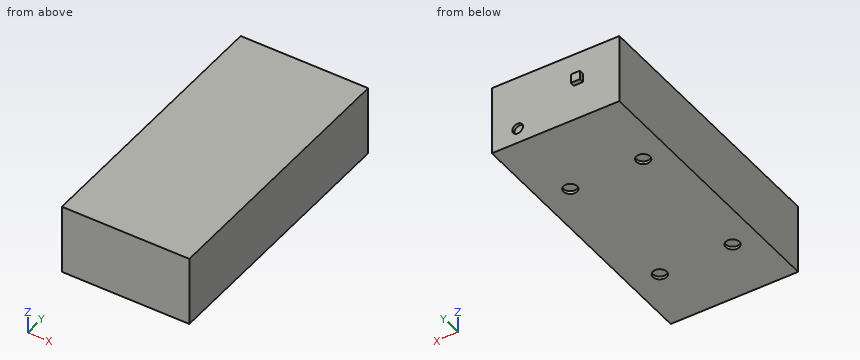
from build123d import *

# Parameters (mm, degrees)
SKETCH1_W           = 90
SKETCH1_H           = 42
SKETCH1_R           = 2.25
BOSS_EXTRUDE1_DEPTH = 23
SKETCH1_3_R         = 2.25
CUT_EXTRUDE1_DEPTH  = 1
SKETCH2_R           = 1.75
CUT_EXTRUDE2_DEPTH  = 1
SKETCH2_3_W         = 3
SKETCH2_3_H         = 3
BOSS_EXTRUDE2_DEPTH = 1.5


with BuildPart() as part:
    # Sketch1 → Boss-Extrude1 (new body)
    # profile 1 of 5: a face of its own
    with BuildSketch(Plane(origin=(0, 0, 0), x_dir=(0, 1, 0), z_dir=(0, 0, 1))):
        Rectangle(SKETCH1_W, SKETCH1_H)
        with Locations((20, 12.5)):
            Circle(SKETCH1_R, mode=Mode.SUBTRACT)
        with Locations((20, -11.5)):
            Circle(SKETCH1_R, mode=Mode.SUBTRACT)
        with Locations((-25, -11.5)):
            Circle(SKETCH1_R, mode=Mode.SUBTRACT)
        with Locations((-25, 12.5)):
            Circle(SKETCH1_R, mode=Mode.SUBTRACT)
    # profile 2 of 5: a face of its own
    with BuildSketch(Plane(origin=(0, 0, 0), x_dir=(0, 1, 0), z_dir=(0, 0, 1))):
        with Locations((-25, -11.5)):
            Circle(SKETCH1_R)
    # profile 3 of 5: a face of its own
    with BuildSketch(Plane(origin=(0, 0, 0), x_dir=(0, 1, 0), z_dir=(0, 0, 1))):
        with Locations((-25, 12.5)):
            Circle(SKETCH1_R)
    # profile 4 of 5: a face of its own
    with BuildSketch(Plane(origin=(0, 0, 0), x_dir=(0, 1, 0), z_dir=(0, 0, 1))):
        with Locations((20, -11.5)):
            Circle(SKETCH1_R)
    # profile 5 of 5: a face of its own
    with BuildSketch(Plane(origin=(0, 0, 0), x_dir=(0, 1, 0), z_dir=(0, 0, 1))):
        with Locations((20, 12.5)):
            Circle(SKETCH1_R)
    extrude(amount=BOSS_EXTRUDE1_DEPTH)

    # Sketch1_3 → Cut-Extrude1 (cut)
    with BuildSketch(Plane(origin=(0, 0, 0), x_dir=(0, 1, 0), z_dir=(0, 0, 1))):
        with Locations(Location((-25, -11.5, 0), (0, 0, 270))):
            Circle(SKETCH1_3_R)
        with Locations(Location((-25, 12.5, 0), (0, 0, 270))):
            Circle(SKETCH1_3_R)
        with Locations(Location((20, -11.5, 0), (0, 0, 270))):
            Circle(SKETCH1_3_R)
        with Locations(Location((20, 12.5, 0), (0, 0, 270))):
            Circle(SKETCH1_3_R)
    extrude(amount=CUT_EXTRUDE1_DEPTH, mode=Mode.SUBTRACT)

    # Sketch2 → Cut-Extrude2 (cut)
    with BuildSketch(Plane(origin=(0, 45, 0), x_dir=(-1, 0, 0), z_dir=(0, 1, 0))):
        with Locations(Location((-12.5, 5, 0), (0, 0, 90))):
            Circle(SKETCH2_R)
    extrude(amount=-CUT_EXTRUDE2_DEPTH, mode=Mode.SUBTRACT)

    # Sketch2_3 → Boss-Extrude2 (add)
    with BuildSketch(Plane(origin=(0, 45, 0), x_dir=(-1, 0, 0), z_dir=(0, 1, 0))):
        with Locations((7.5, 13.5)):
            Rectangle(SKETCH2_3_W, SKETCH2_3_H)
    extrude(amount=BOSS_EXTRUDE2_DEPTH)


solid = part.part
Model file for the job. Use its own axes, mm. Round coordinates to 2 decimals unless told otherwise and drop trailing zeros. Order: outer loops, then holes, each group sorted by start corner. A loop starts at its lowest first (then second) coordinate and runs counter-clockwise, first axis right, second up.
(1) Band-saw the part on B-B (x = -12.5). List the corners of the cut face in (y, z).
(2) Band-saw the part on A-A (z = 13.5). List the corners of the cut face in (x, y).
(3) Band-saw the part on C-C (z = 5). List the corners of the cut face in (x, y).
(4) Band-saw the part on D-D (x = 12.5). List the corners of the cut face in (y, z).
(5) Drill centre lines: line 1 (Y direction, x = -12.5, z = 0.55); line 2 (X direction, y = 44.45, z = 5); line 3 (Y direction, x = -4, z = 3.75). Where is each one in solid material? Low to high.
(6) Pin check, flat tips, straight feed: pin 1 (1.3 mm diameter, centred on x = 12, y = 20, fed in from -Z); pin 2 (6 mm diameter, centred on x = 11.5, y = 20, fed in from -Z); pin 3 (0.8 mm diameter, centred on x = -8, y = 45.5, fed in from +Z); pin 4 (3 mm diameter, centred on x = 3.5, z = 8.5, fed in from +Y). Stop position of each tip, or through.
Verdict:
1. outline: (-45, 0) - (-27.25, 0) - (-27.25, 1) - (-22.75, 1) - (-22.75, 0) - (17.75, 0) - (17.75, 1) - (22.25, 1) - (22.25, 0) - (45, 0) - (45, 23) - (-45, 23) - close
2. outline: (-21, -45) - (21, -45) - (21, 45) - (-6, 45) - (-6, 46.5) - (-9, 46.5) - (-9, 45) - (-21, 45) - close
3. outline: (-21, -45) - (21, -45) - (21, 45) - (14.25, 45) - (14.25, 44) - (10.75, 44) - (10.75, 45) - (-21, 45) - close
4. outline: (-45, 0) - (-27.02, 0) - (-27.02, 1) - (-22.98, 1) - (-22.98, 0) - (17.98, 0) - (17.98, 1) - (22.02, 1) - (22.02, 0) - (45, 0) - (45, 3.25) - (44, 3.25) - (44, 6.75) - (45, 6.75) - (45, 23) - (-45, 23) - close
5. line 1: y = -45 to -27.25, -22.75 to 17.75, 22.25 to 45
5. line 2: x = -21 to 10.75, 14.25 to 21
5. line 3: y = -45 to 45
6. pin 1: stops at z = 1
6. pin 2: stops at z = 0
6. pin 3: stops at z = 15
6. pin 4: stops at y = 45
